Can you work these out from the model? Positions are in its coordinate system, mm. Face numbers are marked on the shaded views. A direction names the side the tool comes from. Coordinates: 2 decimals unless noted, no trailing zeros. Order: outer loops, then holes, each group sorted by start corner. A loop starts at its lowest first (then second) coordinate and runs counter-clockwise, first axis right, second up. Notation, with made-up numbers: (76.25, -17.75) -> (84.25, -17.75) arc R14 ccw to (84.25, -2.75) -> close; hole circle Ø5 at (33.5, -4.5). An arc over 180 degrees is marked (long way). Write item = value, one per line.
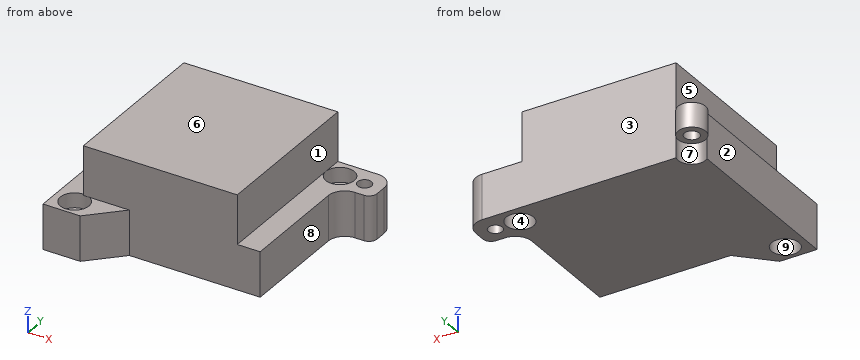
Autodesk Inventor part; units mm, degrees
ref_plane "Arbeitsebene1" through (-9.7716, -9.2098, 6) normal (0, 0, 1) x (1, 0, 0)
ref_plane "YZ Plane" through (0, 0, 0) normal (1, 0, 0) x (0, 1, 0)
ref_plane "XZ Plane" through (0, 0, 0) normal (0, 1, 0) x (-1, 0, 0)
sketch "Skizze1" plane through (0, 0, 0) normal (0, 0, 1) x (1, 0, 0)
  line L0 (14.1792, -17.284) -> (14.1792, 17.716)
  line L1 (14.1792, 17.716) -> (-11.8208, 17.716)
  line L2 (-11.8208, 17.716) -> (-11.8208, -17.284)
  line L3 (-11.8208, -17.284) -> (14.1792, -17.284)
  line L4 (14.1792, -17.284) -> (-11.8208, 17.716) construction
  line L5 (14.1792, 17.716) -> (-11.8208, -17.284) construction
  line L6 (3.4292, 10.341) -> (-6.0708, 10.341) construction
  line L7 (3.4292, 3.091) -> (3.4292, 10.341) construction
  line L8 (-6.0708, 3.091) -> (3.4292, 3.091) construction
  line L9 (-6.0708, 10.341) -> (-6.0708, 3.091) construction
  line L10 (3.4292, 10.341) -> (-6.0708, 3.091) construction
  line L11 (3.4292, 3.091) -> (-6.0708, 10.341) construction
  point P0 (0, 0)
  point P1 (1.1792, 0.216)
  point P2 (1.1792, 0.216)
  point P3 (-1.3208, 6.716)
  point P4 (-1.3208, 6.716)
  point P5 (1.1792, 0.216)
  point P6 (-1.3208, 6.716)
  dimension "d0" = 26
  dimension "d1" = 35
  dimension "d2" = 11
  dimension "d3" = 2.5
sketch "Skizze2" plane through (0, 0, 0) normal (0, 0, 1) x (1, 0, 0)
  line L0 (-3.4208, 1.091) -> (-7.8208, 1.091)
  line L1 (-7.8208, 1.091) -> (-7.8208, 12.341)
  line L2 (-7.8208, 12.341) -> (-3.4208, 12.341)
  line L3 (5.1792, 1.091) -> (0.7792, 1.091)
  line L4 (5.1792, 12.341) -> (5.1792, 1.091)
  line L5 (0.7792, 12.341) -> (5.1792, 12.341)
  circle A0 centre (-9.3002, -4.7384) radius 1.575 construction
  circle A1 centre (11.3792, 14.191) radius 1.575 construction
  circle A2 centre (-9.3002, -4.7384) radius 0.7 construction
  circle A3 centre (-10.7708, 16.016) radius 0.7 construction
  circle A4 centre (11.3792, 14.191) radius 0.7 construction
  line L6 (-3.4208, 12.341) -> (-3.4208, 13.366)
  line L7 (-3.4208, 13.366) -> (0.7792, 13.366)
  line L8 (0.7792, 0.066) -> (-3.4208, 0.066)
  line L9 (-3.4208, 0.066) -> (-3.4208, 1.091)
  line L10 (0.7792, 1.091) -> (0.7792, 0.066)
  line L11 (0.7792, 13.366) -> (0.7792, 12.341)
  line L12 (-12.2708, -9.259) -> (-12.2708, 10.741) construction
  line L13 (14.5292, 16.566) -> (-9.295, 16.566) construction
  arc A5 (16.5292, 14.566) -> (14.5292, 16.566) centre (14.5292, 14.566) ccw
  line L14 (16.5292, 14.566) -> (16.5292, 13.191)
  arc A6 (15.5292, 12.191) -> (16.5292, 13.191) centre (15.5292, 13.191) ccw
  line L15 (15.5292, 12.191) -> (14.4292, 12.191)
  arc A7 (14.4292, 12.191) -> (12.4292, 10.191) centre (14.4292, 10.191) ccw
  line L16 (12.4292, 10.191) -> (12.4292, -3.209)
  line L17 (-3.5708, -3.209) -> (12.4292, -3.209)
  line L18 (-8.1002, -7.7384) -> (-3.5708, -3.209)
  arc A8 (-10.7708, 17.591) -> (-9.295, 16.566) centre (-10.7708, 16.016) ccw construction
  line L19 (-8.1002, -8.7384) -> (-8.1002, -7.7384) construction
  circle A9 centre (-9.3002, -8.7384) radius 0.75 construction
  circle A10 centre (-9.3002, -8.7384) radius 1.2 construction
  line L20 (-10.8208, -7.909) -> (-11.8208, -6.909) construction
  line L21 (-11.8208, -6.909) -> (-11.8208, 14.7109)
  line L22 (-11.8208, -6.909) -> (-10.4976, -8.2322)
  arc A11 (-8.1002, -8.2384) -> (-8.2864, -7.9246) centre (-9.3002, -8.7384) ccw construction
  line L23 (-8.1002, -8.2384) -> (-8.1002, -7.7384) construction
  circle A12 centre (-9.3002, -4.7384) radius 1.675
  circle A13 centre (11.3792, 14.191) radius 1.675
  line L24 (14.5292, 16.566) -> (-9.1887, 16.566)
  arc A14 (-11.8208, 14.7109) -> (-9.1887, 16.566) centre (-10.7708, 16.016) ccw
  circle A15 centre (14.3792, 14.191) radius 0.75 construction
  circle A16 centre (14.3792, 14.191) radius 0.85
  line L25 (-8.1002, -7.7384) -> (-8.2864, -7.9246) construction
  arc A17 (-8.2864, -7.9246) -> (-10.4976, -8.2322) centre (-9.3002, -8.7384) ccw construction
  line L26 (-11.8208, -6.909) -> (-7.2708, -6.909)
  point P0 (0, 0)
  dimension "d4" = 0.1
  dimension "d5" = 0.1
  dimension "d6" = 0.1
  dimension "d7" = 0.1
  dimension "d10" = 0.1
extrude "Extrusion1" add sketch "Skizze2" along normal blind 2.5 contours L0 L1 L2 L6 L7 L11 L5 L4 L3 L10 L8 L9 | L14 A6 L15 A7 L16 L17 L18 L26 L21 A14 L24 A5
sketch "Skizze3" plane through (0, 0, 2.5) normal (0, 0, 1) x (1, 0, 0)
  circle A0 centre (11.3792, 14.191) radius 1.675 construction
  circle A1 centre (-9.3002, -4.7384) radius 1.675 construction
  circle A2 centre (14.3792, 14.191) radius 0.85
  arc A3 (16.5292, 14.566) -> (14.5292, 16.566) centre (14.5292, 14.566) ccw
  line L0 (14.5292, 16.566) -> (-9.1887, 16.566)
  arc A4 (-11.8208, 14.7109) -> (-9.1887, 16.566) centre (-10.7708, 16.016) ccw construction
  line L1 (-11.8208, 14.7109) -> (-11.8208, -6.909)
  line L2 (-7.2708, -6.909) -> (-3.5708, -3.209)
  line L3 (-3.5708, -3.209) -> (12.4292, -3.209)
  line L4 (12.4292, -3.209) -> (12.4292, 10.191)
  arc A5 (14.4292, 12.191) -> (12.4292, 10.191) centre (14.4292, 10.191) ccw
  line L5 (14.4292, 12.191) -> (15.5292, 12.191)
  arc A6 (15.5292, 12.191) -> (16.5292, 13.191) centre (15.5292, 13.191) ccw
  line L6 (16.5292, 13.191) -> (16.5292, 14.566)
  circle A7 centre (11.3792, 14.191) radius 0.7 construction
  circle A8 centre (-9.3002, -4.7384) radius 0.7 construction
  circle A9 centre (-9.3002, -8.7384) radius 0.75 construction
  circle A10 centre (-9.3002, -8.7384) radius 0.85
  line L7 (-8.2864, -7.9246) -> (-3.5708, -3.209)
  arc A11 (-10.4976, -8.2322) -> (-8.2864, -7.9246) centre (-9.3002, -8.7384) ccw
  arc A12 (-9.1887, 16.566) -> (-11.8208, 14.7109) centre (-10.7708, 16.016) ccw
  circle A13 centre (-10.7708, 16.016) radius 0.7 construction
  circle A14 centre (-10.7708, 16.016) radius 0.9
  circle A15 centre (11.3792, 14.191) radius 0.9
  circle A16 centre (-9.3002, -4.7384) radius 0.9
  line L8 (-11.8208, -6.909) -> (-7.2708, -6.909)
  point P0 (0, 0)
  dimension "d11" = 0.1
  dimension "d13" = 1.8
  dimension "d14" = 1.8
  dimension "d15" = 1.8
ref_plane "Arbeitsebene1" through (-9.7716, -9.2098, 6) normal (0, 0, 1) x (1, 0, 0)
extrude "Extrusion2" add sketch "Skizze3" along normal blind 3 contours L6 A6 L5 A5 L4 L3 L2 L8 L1 A12 L0 A3
sketch "Skizze4" plane through (-9.1887, 16.566, 5.5) normal (0, 0, 1) x (1, 0, 0)
  circle A0 centre (-0.1115, -21.3043) radius 0.7 construction
  circle A1 centre (-1.5821, -0.55) radius 0.7 construction
  circle A2 centre (20.5679, -2.375) radius 0.7 construction
  point P0 (9.1887, -16.566)
hole "Bohrung1" at (-9.3002, -4.7384, 5.5) at (11.3792, 14.191, 5.5) direction (0, 0, -1) diameter 1.8 end through all counterbore diameter 3.5 counterbore depth 1.8
sketch "Sketch8" plane through (0, 0, 5.5) normal (0, 0, 1) x (1, 0, 0)
  circle A0 centre (-9.3002, -4.7384) radius 1.75
  circle A1 centre (11.3792, 14.191) radius 1.75
  circle A2 centre (-10.7708, 16.016) radius 0.9
  circle A3 centre (14.3792, 14.191) radius 0.85
  arc A4 (16.5292, 14.566) -> (14.5292, 16.566) centre (14.5292, 14.566) ccw
  line L0 (14.5292, 16.566) -> (-9.1887, 16.566)
  arc A5 (-9.1887, 16.566) -> (-11.8208, 14.7109) centre (-10.7708, 16.016) ccw
  line L1 (-11.8208, 14.7109) -> (-11.8208, -6.909)
  line L2 (-11.8208, -6.909) -> (-7.2708, -6.909)
  line L3 (-7.2708, -6.909) -> (-3.5708, -3.209)
  line L4 (-3.5708, -3.209) -> (12.4292, -3.209)
  line L5 (12.4292, -3.209) -> (12.4292, 10.191)
  arc A6 (14.4292, 12.191) -> (12.4292, 10.191) centre (14.4292, 10.191) ccw
  line L6 (14.4292, 12.191) -> (15.5292, 12.191)
  arc A7 (15.5292, 12.191) -> (16.5292, 13.191) centre (15.5292, 13.191) ccw
  line L7 (16.5292, 13.191) -> (16.5292, 14.566)
  line L8 (12.4292, -3.209) -> (-3.5708, -3.209)
  line L9 (-9.1887, 16.566) -> (14.5292, 16.566)
  line L10 (9.6292, -3.209) -> (-9.1887, -3.209)
  line L11 (-9.1887, -3.209) -> (-9.1887, 16.566)
  line L12 (-9.1887, 16.566) -> (9.6292, 16.566)
  line L13 (9.6292, 16.566) -> (9.6292, -3.209)
  circle A8 centre (11.3792, 14.191) radius 1.75
  point P0 (0, 0)
extrude "Extrusion6" add sketch "Sketch8" along normal blind 6 contours L10 L11 A0 | A0 L11 L0 L13 L4 L10 picked at (-8.7742, -3.1728)
properties part number "Raman2Go_Adapterplatte2_XY-TischChina"
Item 1: For the marked faces 1, 2, 3, 4 and 5, which set-ups out of +Z, -Z, +X, -X, +Y, -Y let a thin tool reach every point of the face, with its end or its side?
A:
face_1 = +Z, +X, +Y, -Y
face_2 = +Z, -Z, -X, -Y
face_3 = +Z, -Z, +X, +Y
face_4 = -Z
face_5 = +Z, -X, +Y, -Y
Item 2: I want a section at D-D, the plane x = 3.75. Please give me the cut outline in (y, z).
A:
outline = (-3.21, 0) -> (16.57, 0) -> (16.57, 11.5) -> (-3.21, 11.5) -> close
Item 3: I want a section at A-A, the plane x = 14. Please give me the cut outline in (y, z).
A:
outline = (12.14, 0) -> (13.43, 0) -> (13.43, 5.5) -> (12.14, 5.5) -> close; (14.95, 0) -> (16.57, 0) -> (16.57, 5.5) -> (14.95, 5.5) -> close
Item 4: I'm going to push flat-ended pins straight in: P1, Ø2, axis at x = -9.3, y = -4.74, coming from the -Z side; P2, Ø0.9, axis at x = 15, z = 3.5, coming from the -Y side; P3, Ø6, axis at x = 3, z = 6.5, coming from the +Y side. Where does each tip first touch, or does it pass through?
A:
P1 = 2.5
P2 = 12.19
P3 = 16.57
Item 5: If I drill on probe 1 along X at (y, z) = (-0.75, 7.25); probe 2 along Y at (x, z) = (-0.5, 6); probe 3 along Y at (x, z) = (14.5, 1.5), over which ranges is the centre line in solid material (lowest first)?
A:
probe_1 = -9.19 to 9.63
probe_2 = -3.21 to 16.57
probe_3 = 12.19 to 13.35, 15.03 to 16.57
Item 6: If we mould it in two halves opening along X, with no side actions, what happens to the marked faces 6, 7, 8 and 9? For each: pulls with the +X half, pulls with the -X half, needs draft (parallel to the pull), parting line crosses it, or undercut.
A:
face_6 = needs draft
face_7 = undercut
face_8 = pulls with the +X half
face_9 = undercut
Item 7: I want a section at B-B, the plane y = -0.25. Please give me the cut outline in (x, z), plus the area to 3 significant figures.
A:
outline = (-11.82, 0) -> (12.43, 0) -> (12.43, 5.5) -> (9.63, 5.5) -> (9.63, 11.5) -> (-9.19, 11.5) -> (-9.19, 5.5) -> (-11.82, 5.5) -> close
area = 246 mm2
Item 8: I want a section at C-C, the plane z = 7.25. Please give me the cut outline in (x, y).
A:
outline = (-9.19, -3.21) -> (9.63, -3.21) -> (9.63, 16.57) -> (-9.19, 16.57) -> close
